Part model, mm, in its own coordinate system. A direction names the side the tool comes from. Round coordinates to 2 decimals unless told otherwise and drop trailing zeros. Write each loop counter-clockwise with the first axis right and the second up, starting at its lowest first coordinate (ties: lowest second). Pieces come first, ordered by that corner, then holes. Notation, with made-up numbers: (45, -5.75) -> (89, -5.75) arc R23 ccw to (89, 4.25) -> close; hole circle Ø9 at (-23.75, 6.25). An arc over 180 degrees is marked (long way). Return JSON: item names as keys, results as strings. Group by question number.
(1) Mould opens along Z. For faces 1 (the cylindrical face through (44.71, 31.8, 4)), 2 (the flat face through (-29, -28, 3)), 3 (the cylindrical face through (-40.208, 16.586, 6.084)) say: +Z half, -Z half, draft (parallel to the pull), parting line (faces both ways), or undercut.
(2) Saw through at A-A (y = 26.87). List the corners of the cut face in (x, z).
(3) Drop flat-ended pins along their axis: pin 1 Ø10 at (x, y) = (-28.5, -28.5) entering from -Z; pin 2 Ø5 at (x, z) = (34.5, 6.5) entering from -Y; pin 3 Ø2.5 at (x, y) = (28.5, 26.5) entering from -Z; pin 4 Ø3.5 at (x, y) = (40, 15) entering from +Z. Give the stop position or say it passes through.
(4) Tool access for faces 4 (the cylindrical face through (44.71, -31.8, 11)), 5 (the cylindrical face through (-44.71, 31.8, 4)), 6 (the flat face through (-0.616, -31.929, 10.715)), 7 (the cylindrical face through (42.4, 16.8, 13.5)), 8 (the cylindrical face through (27.46, 31.33, 1.48)): list every direction of +Z, -Z, +X, -X, +Y, -Y with a clear straight run to the whole face (end or side of a thin tool).
(5) Saw through at B-B (x = -40). List the corners of the cut face in (y, z).
(6) Saw through at C-C (x = -20.5). List the corners of the cut face in (y, z).
(7) Saw through at D-D (y = 15). List the corners of the cut face in (x, z).
(8) Drill centre lines: L1, parallel to X at y = -26.87, z = 9; L2, parallel to X at y = -26.5, z = 2.75; L3, parallel to Y at x = -40, z = 3.25. Where is each one in solid material? Low to high. Write a range as from..to.
from build123d import *

# Parameters (mm, degrees)
SKETCH_1_W          = 90
SKETCH_1_H          = 73
SKETCH_1_R          = 2.1
EXTRUDE_1_DEPTH     = 15
SKETCH_2_R          = 4.5
CUT_EXTRUDE_1_DEPTH = 3
CUT_EXTRUDE_4_DEPTH = 99.271308122
SKETCH_6_R          = 1.6
CUT_EXTRUDE_5_DEPTH = 60.851900555
SKETCH_7_R          = 3
CUT_EXTRUDE_6_DEPTH = 3
FILLET_5_R          = 1
FILLET_6_R          = 1
FILLET_7_R          = 1
FILLET_8_R          = 1


with BuildPart() as part:
    # 草图1 → 凸台-拉伸1 (new body)
    with BuildSketch(Plane.XY):
        Rectangle(SKETCH_1_W, SKETCH_1_H)
        with Locations((-26.87, 26.87)):
            Circle(SKETCH_1_R, mode=Mode.SUBTRACT)
        with Locations(Location((26.87, 26.87, 0), (0, 0, 180))):
            Circle(SKETCH_1_R, mode=Mode.SUBTRACT)
        with Locations((26.87, -26.87)):
            Circle(SKETCH_1_R, mode=Mode.SUBTRACT)
        with Locations(Location((-26.87, -26.87, 0), (0, 0, 180))):
            Circle(SKETCH_1_R, mode=Mode.SUBTRACT)
    extrude(amount=EXTRUDE_1_DEPTH)

    # 草图2 → 切除-拉伸1 (cut)
    with BuildSketch(Plane(origin=(0, 0, 0), x_dir=(-1, 0, 0), z_dir=(0, 0, -1))):
        with Locations((-26.87, 26.87)):
            Circle(SKETCH_2_R)
        with Locations(Location((26.87, 26.87, 0), (0, 0, 180))):
            Circle(SKETCH_2_R)
        with Locations((26.87, -26.87)):
            Circle(SKETCH_2_R)
        with Locations(Location((-26.87, -26.87, 0), (0, 0, 180))):
            Circle(SKETCH_2_R)
    extrude(amount=-CUT_EXTRUDE_1_DEPTH, mode=Mode.SUBTRACT)

    # 草图5 → 切除-拉伸4 (cut, through all)
    with BuildSketch(Plane.ZY.offset(45)):
        Polygon((0, 36.5), (7.5, 28.5), (15, 36.5), align=None)
        Polygon((0, -36.5), (7.5, -28.5), (15, -36.5), align=None)
    extrude(amount=-CUT_EXTRUDE_4_DEPTH, mode=Mode.SUBTRACT)

    # 草图6 → 切除-拉伸5 (cut, through all)
    with BuildSketch(Plane.XY.offset(15)):
        with Locations((-40, 15)):
            Circle(SKETCH_6_R)
        with Locations(Location((-40, -15, 0), (0, 0, 180))):
            Circle(SKETCH_6_R)
        with Locations((40, -15)):
            Circle(SKETCH_6_R)
        with Locations(Location((40, 15, 0), (0, 0, 180))):
            Circle(SKETCH_6_R)
    extrude(amount=-CUT_EXTRUDE_5_DEPTH, mode=Mode.SUBTRACT)

    # 草图7 → 切除-拉伸6 (cut)
    with BuildSketch(Plane.XY.offset(15)):
        with Locations((-40, 15)):
            Circle(SKETCH_7_R)
        with Locations(Location((-40, -15, 0), (0, 0, 180))):
            Circle(SKETCH_7_R)
        with Locations((40, -15)):
            Circle(SKETCH_7_R)
        with Locations(Location((40, 15, 0), (0, 0, 180))):
            Circle(SKETCH_7_R)
    extrude(amount=-CUT_EXTRUDE_6_DEPTH, mode=Mode.SUBTRACT)

    # 圆角5
    # the kernel refuses this fillet: 1 mm, written as the material it adds along each edge
    with BuildSketch(Plane(origin=(-45, -28.5, 7.5), x_dir=(0, -0.7295372041400846, -0.6839411288813302), z_dir=(1, 0, 0))) as fillet_5_piece_1_section:
        with BuildLine():
            CenterArc((FILLET_5_R * 1.06666666667, -FILLET_5_R), FILLET_5_R, 90, 93.695220532)
            Line((FILLET_5_R * 0.0687456687457, -FILLET_5_R * 1.06444906445), (0, 0))
            Line((0, 0), (FILLET_5_R * 1.06666666667, 0))
        make_face()
    fillet_5_piece_1 = extrude(amount=19.47261984, mode=Mode.PRIVATE)
    fillet_5_piece_1 = fillet_5_piece_1 - Plane(origin=(-26.87, -26.87, 7.500000002), x_dir=(-1, 0, 0), z_dir=(0, 0, -1)) * Cylinder(2.1, 44, mode=Mode.PRIVATE)
    add(fillet_5_piece_1)
    with BuildSketch(Plane(origin=(25.52738016, -28.5, 7.5), x_dir=(0, -0.7295372041400846, -0.6839411288813302), z_dir=(1, 0, 0))) as fillet_5_piece_2_section:
        with BuildLine():
            CenterArc((FILLET_5_R * 1.06666666667, -FILLET_5_R), FILLET_5_R, 90, 93.695220532)
            Line((FILLET_5_R * 0.0687456687457, -FILLET_5_R * 1.06444906445), (0, 0))
            Line((0, 0), (FILLET_5_R * 1.06666666667, 0))
        make_face()
    fillet_5_piece_2 = extrude(amount=19.47261984, mode=Mode.PRIVATE)
    fillet_5_piece_2 = fillet_5_piece_2 - Plane(origin=(26.87, -26.87, 7.500000002), x_dir=(1, 0, 0), z_dir=(0, 0, -1)) * Cylinder(2.1, 44, mode=Mode.PRIVATE)
    add(fillet_5_piece_2)
    with BuildSketch(Plane(origin=(-28.21261984, -28.5, 7.5), x_dir=(0, -0.7295372041400846, -0.6839411288813302), z_dir=(1, 0, 0))) as fillet_5_piece_3_section:
        with BuildLine():
            CenterArc((FILLET_5_R * 1.06666666667, -FILLET_5_R), FILLET_5_R, 90, 93.695220532)
            Line((FILLET_5_R * 0.0687456687457, -FILLET_5_R * 1.06444906445), (0, 0))
            Line((0, 0), (FILLET_5_R * 1.06666666667, 0))
        make_face()
    fillet_5_piece_3 = extrude(amount=56.425239679, mode=Mode.PRIVATE)
    fillet_5_piece_3 = fillet_5_piece_3 - Plane(origin=(-26.87, -26.87, 7.500000001), x_dir=(-1, 0, 0), z_dir=(0, 0, -1)) * Cylinder(2.1, 118, mode=Mode.PRIVATE)
    fillet_5_piece_3 = fillet_5_piece_3 - Plane(origin=(26.87, -26.87, 7.500000001), x_dir=(1, 0, 0), z_dir=(0, 0, -1)) * Cylinder(2.1, 118, mode=Mode.PRIVATE)
    add(fillet_5_piece_3)
    # the kernel refuses this fillet: 1 mm, written as the material it takes off along each edge
    with BuildSketch(Plane(origin=(51.321952033, -36.5, 15), x_dir=(0, 1, 0), z_dir=(-1, 0, 0))) as fillet_5_2_piece_1:
        with BuildLine():
            CenterArc((FILLET_5_R * 2.5287808133, FILLET_5_R), FILLET_5_R, 133.152389734, 136.847610266)
            Line((FILLET_5_R * 1.84483968442, FILLET_5_R * 1.72953720414), (0, 0))
            Line((0, 0), (FILLET_5_R * 2.5287808133, 0))
        make_face()
    extrude(amount=102.643904066, mode=Mode.SUBTRACT)
    with BuildSketch(Plane(origin=(51.321952033, -36.5, 0), x_dir=(0, 1, 0), z_dir=(-1, 0, 0))) as fillet_5_2_piece_2:
        with BuildLine():
            CenterArc((FILLET_5_R * 2.5287808133, -FILLET_5_R), FILLET_5_R, 90, 136.847610266)
            Line((FILLET_5_R * 1.84483968442, -FILLET_5_R * 1.72953720414), (0, 0))
            Line((0, 0), (FILLET_5_R * 2.5287808133, 0))
        make_face()
    extrude(amount=102.643904066, mode=Mode.SUBTRACT)

    # 圆角6
    # the kernel refuses this fillet: 1 mm, written as the material it adds along each edge
    with BuildSketch(Plane(origin=(-28.21261984, 28.5, 7.5), x_dir=(0, 0.729537204140085, -0.6839411288813297), z_dir=(1, 0, 0))) as fillet_6_piece_1_section:
        with BuildLine():
            CenterArc((FILLET_6_R * 1.06666666667, FILLET_6_R), FILLET_6_R, 176.304779468, 93.695220532)
            Line((FILLET_6_R * 0.0687456687457, FILLET_6_R * 1.06444906445), (0, 0))
            Line((0, 0), (FILLET_6_R * 1.06666666667, 0))
        make_face()
    fillet_6_piece_1 = extrude(amount=56.425239679, mode=Mode.PRIVATE)
    fillet_6_piece_1 = fillet_6_piece_1 - Plane(origin=(-26.87, 26.87, 7.499999974), x_dir=(1, 0, 0), z_dir=(0, 0, -1)) * Cylinder(2.1, 118, mode=Mode.PRIVATE)
    fillet_6_piece_1 = fillet_6_piece_1 - Plane(origin=(26.87, 26.87, 7.499999974), x_dir=(-1, 0, 0), z_dir=(0, 0, -1)) * Cylinder(2.1, 118, mode=Mode.PRIVATE)
    add(fillet_6_piece_1)
    with BuildSketch(Plane(origin=(-45, 28.5, 7.5), x_dir=(0, 0.7295372041400854, -0.6839411288813294), z_dir=(1, 0, 0))) as fillet_6_piece_2_section:
        with BuildLine():
            CenterArc((FILLET_6_R * 1.06666666667, FILLET_6_R), FILLET_6_R, 176.304779468, 93.695220532)
            Line((FILLET_6_R * 0.0687456687457, FILLET_6_R * 1.06444906445), (0, 0))
            Line((0, 0), (FILLET_6_R * 1.06666666667, 0))
        make_face()
    fillet_6_piece_2 = extrude(amount=19.47261984, mode=Mode.PRIVATE)
    fillet_6_piece_2 = fillet_6_piece_2 - Plane(origin=(-26.87, 26.87, 7.500000011), x_dir=(1, 0, 0), z_dir=(0, 0, -1)) * Cylinder(2.1, 44, mode=Mode.PRIVATE)
    add(fillet_6_piece_2)
    with BuildSketch(Plane(origin=(25.52738016, 28.5, 7.5), x_dir=(0, 0.729537204140085, -0.6839411288813297), z_dir=(1, 0, 0))) as fillet_6_piece_3_section:
        with BuildLine():
            CenterArc((FILLET_6_R * 1.06666666667, FILLET_6_R), FILLET_6_R, 176.304779468, 93.695220532)
            Line((FILLET_6_R * 0.0687456687457, FILLET_6_R * 1.06444906445), (0, 0))
            Line((0, 0), (FILLET_6_R * 1.06666666667, 0))
        make_face()
    fillet_6_piece_3 = extrude(amount=19.47261984, mode=Mode.PRIVATE)
    fillet_6_piece_3 = fillet_6_piece_3 - Plane(origin=(26.87, 26.87, 7.500000017), x_dir=(-1, 0, 0), z_dir=(0, 0, -1)) * Cylinder(2.1, 44, mode=Mode.PRIVATE)
    add(fillet_6_piece_3)
    # the kernel refuses this fillet: 1 mm, written as the material it takes off along each edge
    with BuildSketch(Plane(origin=(-51.321952033, 36.5, 0), x_dir=(0, -1, 0), z_dir=(1, 0, 0)), Plane(origin=(-51.321952033, 36.5, 15), x_dir=(0, -0.7295372041400834, -0.6839411288813316), z_dir=(1, 0, 0))) as fillet_6_2_piece_1:
        with BuildLine():
            CenterArc((FILLET_6_R * 2.5287808133, -FILLET_6_R), FILLET_6_R, 90, 136.847610266)
            Line((FILLET_6_R * 1.84483968442, -FILLET_6_R * 1.72953720414), (0, 0))
            Line((0, 0), (FILLET_6_R * 2.5287808133, 0))
        make_face()
    extrude(amount=102.643904066, mode=Mode.SUBTRACT)

    # 圆角7
    fillet_7_edges = [part.edges().sort_by_distance(p)[0] for p in [
        (45, -31.966666667, 4.25),
        (45, 0, 15),
        (45, -31.966666667, 10.75),
        (45, 0, 0),
        (45, -34.90114854, 14.367738219),
        (45, -34.90114854, 0.632261781),
        (45, -28.962114147, 7.5),
        (45, 31.966666667, 4.25),
        (45, 31.966666667, 10.75),
        (45, 34.90114854, 14.367738219),
        (45, 34.90114854, 0.632261781),
        (45, 28.962114147, 7.5),
    ]]
    fillet(fillet_7_edges, radius=FILLET_7_R)

    # 圆角8
    fillet_8_edges = [part.edges().sort_by_distance(p)[0] for p in [
        (-45, -31.966666667, 4.25),
        (-45, -31.966666667, 10.75),
        (-45, -34.90114854, 14.367738219),
        (-45, -34.90114854, 0.632261781),
        (-45, -28.962114147, 7.5),
        (-45, 31.966666667, 4.25),
        (-45, 0, 0),
        (-45, 0, 15),
        (-45, 31.966666667, 10.75),
        (-45, 34.90114854, 14.367738219),
        (-45, 34.90114854, 0.632261781),
        (-45, 28.962114147, 7.5),
    ]]
    fillet(fillet_8_edges, radius=FILLET_8_R)


solid = part.part
Computed values:
{
 "1": {"face 1": "undercut", "face 2": "-Z half", "face 3": "draft"},
 "2": {"outline": "(-45, 1) arc R1 ccw to (-44, 0) -> (-31.37, 0) -> (-31.37, 3) -> (-28.97, 3) -> (-28.97, 15) -> (-44, 15) arc R1 ccw to (-45, 14) -> close; (-24.77, 3) -> (-22.37, 3) -> (-22.37, 0) -> (22.37, 0) -> (22.37, 3) -> (24.77, 3) -> (24.77, 15) -> (-24.77, 15) -> close; (28.97, 3) -> (31.37, 3) -> (31.37, 0) -> (44, 0) arc R1 ccw to (45, 1) -> (45, 14) arc R1 ccw to (44, 15) -> (28.97, 15) -> close"},
 "3": {"pin 1": "z = 0", "pin 2": "y = -32.23", "pin 3": "z = 3", "pin 4": "z = 12"},
 "4": {"face 4": "+X, -Y", "face 5": "-X, +Y", "face 6": "+X, -X, -Y", "face 7": "+Z", "face 8": "-Z"},
 "5": {"outline": "(-34.66, 1.73) arc R1 ccw to (-33.97, 0) -> (-16.6, 0) -> (-16.6, 12) -> (-18, 12) -> (-18, 15) -> (-33.97, 15) arc R1 ccw to (-34.66, 13.27) -> (-29.28, 8.23) arc R1 cw to (-29.28, 6.77) -> close; (-13.4, 0) -> (13.4, 0) -> (13.4, 12) -> (12, 12) -> (12, 15) -> (-12, 15) -> (-12, 12) -> (-13.4, 12) -> close; (16.6, 0) -> (33.97, 0) arc R1 ccw to (34.66, 1.73) -> (29.28, 6.77) arc R1 cw to (29.28, 8.23) -> (34.66, 13.27) arc R1 ccw to (33.97, 15) -> (18, 15) -> (18, 12) -> (16.6, 12) -> close"},
 "6": {"outline": "(-34.66, 1.73) arc R1 ccw to (-33.97, 0) -> (33.97, 0) arc R1 ccw to (34.66, 1.73) -> (29.28, 6.77) arc R1 cw to (29.28, 8.23) -> (34.66, 13.27) arc R1 ccw to (33.97, 15) -> (-33.97, 15) arc R1 ccw to (-34.66, 13.27) -> (-29.28, 8.23) arc R1 cw to (-29.28, 6.77) -> close"},
 "7": {"outline": "(-45, 1) arc R1 ccw to (-44, 0) -> (-41.6, 0) -> (-41.6, 12) -> (-43, 12) -> (-43, 15) -> (-44, 15) arc R1 ccw to (-45, 14) -> close; (-38.4, 0) -> (38.4, 0) -> (38.4, 12) -> (37, 12) -> (37, 15) -> (-37, 15) -> (-37, 12) -> (-38.4, 12) -> close; (41.6, 0) -> (44, 0) arc R1 ccw to (45, 1) -> (45, 14) arc R1 ccw to (44, 15) -> (43, 15) -> (43, 12) -> (41.6, 12) -> close"},
 "8": {"L1": "-45..-28.97, -24.77..24.77, 28.97..45", "L2": "-45..-31.35, -22.39..22.39, 31.35..45", "L3": "-33.03..-16.6, -13.4..13.4, 16.6..33.03"}
}
